from build123d import *

# Parameters (mm, degrees)
IZIM1_W                     = 122
IZIM1_H                     = 30
Y_KSEKLIK_EKSTR_ZYON1_DEPTH = 46.7
IZIM2_W                     = 38
IZIM2_H                     = 30
Y_KSEKLIK_EKSTR_ZYON2_DEPTH = 1
IZIM3_R                     = 2.5
KES_EKSTR_ZYON1_DEPTH       = 20
KES_EKSTR_ZYON2_DEPTH       = 38
IZIM5_R                     = 10
KES_EKSTR_ZYON3_DEPTH       = 38
Y_KSEKLIK_EKSTR_ZYON3_DEPTH = 14.5
IZIM7_R                     = 9
Y_KSEKLIK_EKSTR_ZYON4_DEPTH = 15
IZIM8_W                     = 38
IZIM8_H                     = 30
Y_KSEKLIK_EKSTR_ZYON5_DEPTH = 1
IZIM9_R                     = 2.5
KES_EKSTR_ZYON4_DEPTH       = 20
Y_KSEKLIK_EKSTR_ZYON6_DEPTH = 10
IZIM11_R                    = 3
Y_KSEKLIK_EKSTR_ZYON7_DEPTH = 20


with BuildPart() as part:
    # Çizim1 → Yükseklik-Ekstrüzyon1 (new body)
    with BuildSketch(Plane.XY):
        Rectangle(IZIM1_W, IZIM1_H)
    extrude(amount=Y_KSEKLIK_EKSTR_ZYON1_DEPTH)

    # Çizim2 → Yükseklik-Ekstrüzyon2 (add)
    with BuildSketch(Plane(origin=(0, 0, 0), x_dir=(-1, 0, 0), z_dir=(0, 0, -1))):
        with Locations((-42, 0)):
            Rectangle(IZIM2_W, IZIM2_H)
    extrude(amount=Y_KSEKLIK_EKSTR_ZYON2_DEPTH)

    # Çizim3 → Kes-Ekstrüzyon1 (cut)
    with BuildSketch(Plane(origin=(0, 0, -1), x_dir=(-1, 0, 0), z_dir=(0, 0, -1))):
        with Locations((-29, 7.5)):
            Circle(IZIM3_R)
        with Locations((-44, 7.5)):
            Circle(IZIM3_R)
        with Locations((-44, -7.5)):
            Circle(IZIM3_R)
        with Locations((-29, -7.5)):
            Circle(IZIM3_R)
    extrude(amount=-KES_EKSTR_ZYON1_DEPTH, mode=Mode.SUBTRACT)

    # Çizim4 → Kes-Ekstrüzyon2 (cut)
    with BuildSketch(Plane.XZ.offset(15)):
        with BuildLine():
            Line((13.5, 6.27), (-22.5, 6.27))
            Line((-22.5, 6.27), (-22.5, 20.35))
            Line((-22.5, 20.35), (-17.149110641, 20.35))
            ThreePointArc((-17.149110641, 20.35), (-4.5, 10.35), (8.149110641, 20.35))
            Line((8.149110641, 20.35), (13.5, 20.35))
            Line((13.5, 20.35), (13.5, 6.27))
        make_face()
        with BuildLine():
            Line((13.5, 40.43), (-22.5, 40.43))
            Line((-22.5, 40.43), (-22.5, 26.35))
            Line((-22.5, 26.35), (-17.149110641, 26.35))
            ThreePointArc((-17.149110641, 26.35), (-4.5, 36.35), (8.149110641, 26.35))
            Line((8.149110641, 26.35), (13.5, 26.35))
            Line((13.5, 26.35), (13.5, 40.43))
        make_face()
    extrude(amount=-KES_EKSTR_ZYON2_DEPTH, mode=Mode.SUBTRACT)

    # Çizim5 → Kes-Ekstrüzyon3 (cut)
    with BuildSketch(Plane.XZ.offset(15)):
        with Locations(Location((-4.5, 23.35, 0), (0, 0, 270))):
            Circle(IZIM5_R)
    extrude(amount=-KES_EKSTR_ZYON3_DEPTH, mode=Mode.SUBTRACT)

    # Çizim6 → Yükseklik-Ekstrüzyon3 (add)
    with BuildSketch(Plane.ZY.offset(61)):
        Polygon((26, 12.701705922), (15, 6.350852961), (15, -6.350852961), (26, -12.701705922), (37, -6.350852961), (37, 6.350852961), align=None)
    extrude(amount=Y_KSEKLIK_EKSTR_ZYON3_DEPTH)

    # Çizim7 → Yükseklik-Ekstrüzyon4 (add)
    with BuildSketch(Plane.ZY.offset(75.5)):
        with Locations((26, 0)):
            Circle(IZIM7_R)
    extrude(amount=Y_KSEKLIK_EKSTR_ZYON4_DEPTH)

    # Çizim8 → Yükseklik-Ekstrüzyon5 (add)
    with BuildSketch(Plane.XY.offset(46.7)):
        with Locations((-42, 0)):
            Rectangle(IZIM8_W, IZIM8_H)
    extrude(amount=Y_KSEKLIK_EKSTR_ZYON5_DEPTH)

    # Çizim9 → Kes-Ekstrüzyon4 (cut)
    with BuildSketch(Plane.XY.offset(47.7)):
        with Locations((-45.2, 7.5)):
            Circle(IZIM9_R)
        with Locations((-45.2, -7.5)):
            Circle(IZIM9_R)
        with Locations((-30.2, -7.5)):
            Circle(IZIM9_R)
        with Locations((-30.2, 7.5)):
            Circle(IZIM9_R)
    extrude(amount=-KES_EKSTR_ZYON4_DEPTH, mode=Mode.SUBTRACT)

    # Çizim10 → Yükseklik-Ekstrüzyon6 (add)
    with BuildSketch(Plane.ZY.offset(90.5)):
        Polygon((26, 10.392304845), (17, 5.196152423), (17, -5.196152423), (26, -10.392304845), (35, -5.196152423), (35, 5.196152423), align=None)
    extrude(amount=Y_KSEKLIK_EKSTR_ZYON6_DEPTH)

    # Çizim11 → Yükseklik-Ekstrüzyon7 (add)
    with BuildSketch(Plane.ZY.offset(100.5)):
        with Locations((26, 0)):
            Circle(IZIM11_R)
    extrude(amount=Y_KSEKLIK_EKSTR_ZYON7_DEPTH)


solid = part.part
Model file for the job. Use its own axes, mm. A direction names the side the tool comes from. Round coordinates to 2 decimals unless told otherwise and drop trailing zeros. Loops run counter-clockwise (first coordinate to the right, second up) from the corner with the lowest first, then second, coordinate; pieces in that order, holes last.
1. Band-saw the part on D-D, the plane x = -41. List the corners of the cut face in (y, z), and give its area (3 significant figures).
Check values:
outline: (-15, 0) - (15, 0) - (15, 47.7) - (-15, 47.7) - close
area: 1,430 mm2
2. Drop flat-ended pins along their axis: P1, Ø9, axis at x = -7, y = 4, coming from the +Z side; P2, Ø1.5, axis at x = -29.5, y = -7.5, coming from the +Z side; P3, Ø4.5, axis at x = 44, y = -7.5, coming from the -Z side. Give the stop position or say it passes through.
Check values:
P1: stops at z = 46.7
P2: stops at z = 27.7
P3: stops at z = 19
3. Mould opens along Y. For faces 1 (the cylindrical face through (-47.7, -7.4, 37.8)), 2 (the flat face through (11, 0, 26.35)), 3 (the flat face through (-1, 15, 12)) say: +Y half, -Y half, draft (parallel to the pull), parting line (faces both ways), or undercut.
Check values:
face 1: undercut
face 2: draft
face 3: +Y half
4. Tool access for faces 4 (the flat face through (-95, 0, 35)), 5 (the flat face through (11, 0, 20.35)), 6 (the flat face through (44, -7, 19)), 7 (the flat face through (-68.148, 9.571, 20.577)), 8 (the flat face through (-68.15, -9.48, 20.42)): list every direction of +Z, -Z, +X, -X, +Y, -Y with a clear straight run to the whole face (end or side of a thin tool).
Check values:
face 4: +Z, -X, +Y, -Y
face 5: +Y, -Y
face 6: -Z
face 7: -Z, -X, +Y
face 8: -Z, -X, -Y
5. Band-saw the part on B-B, the plane x = 0. List the corners of the cut face in (y, z).
Check values:
outline: (-15, 0) - (15, 0) - (15, 6.27) - (-15, 6.27) - close; (-15, 11.15) - (15, 11.15) - (15, 14.42) - (-15, 14.42) - close; (-15, 32.28) - (15, 32.28) - (15, 35.55) - (-15, 35.55) - close; (-15, 40.43) - (15, 40.43) - (15, 46.7) - (-15, 46.7) - close
6. Band-saw the part on A-A, the plane z = 42.5. List the corners of the cut face in (x, y), and give its area (3 significant figures).
Check values:
outline: (-61, -15) - (61, -15) - (61, 15) - (-61, 15) - close; hole circle Ø5 at (-45.2, -7.5); hole circle Ø5 at (-45.2, 7.5); hole circle Ø5 at (-30.2, -7.5); hole circle Ø5 at (-30.2, 7.5)
area: 3,580 mm2
7. Band-saw the part on C-C, the plane x = 44. List the corners of the cut face in (y, z), and give its area (3 significant figures).
Check values:
outline: (-15, -1) - (-10, -1) - (-10, 19) - (-5, 19) - (-5, -1) - (5, -1) - (5, 19) - (10, 19) - (10, -1) - (15, -1) - (15, 46.7) - (-15, 46.7) - close
area: 1,230 mm2
8. Wall check: probe 1 along Y at (x, z) = (-45.2, 43.5); probe 2 along Z at (x, y) = (-21.5, -8); probe 3 along X at (y, z) = (-6.5, 23.35). Give the ranges that are in metal, low to high.
Check values:
probe 1: y = -15 to -10, -5 to 5, 10 to 15
probe 2: z = 0 to 6.27, 20.35 to 26.35, 40.43 to 46.7
probe 3: x = -100.5 to -14.5, 5.5 to 61
